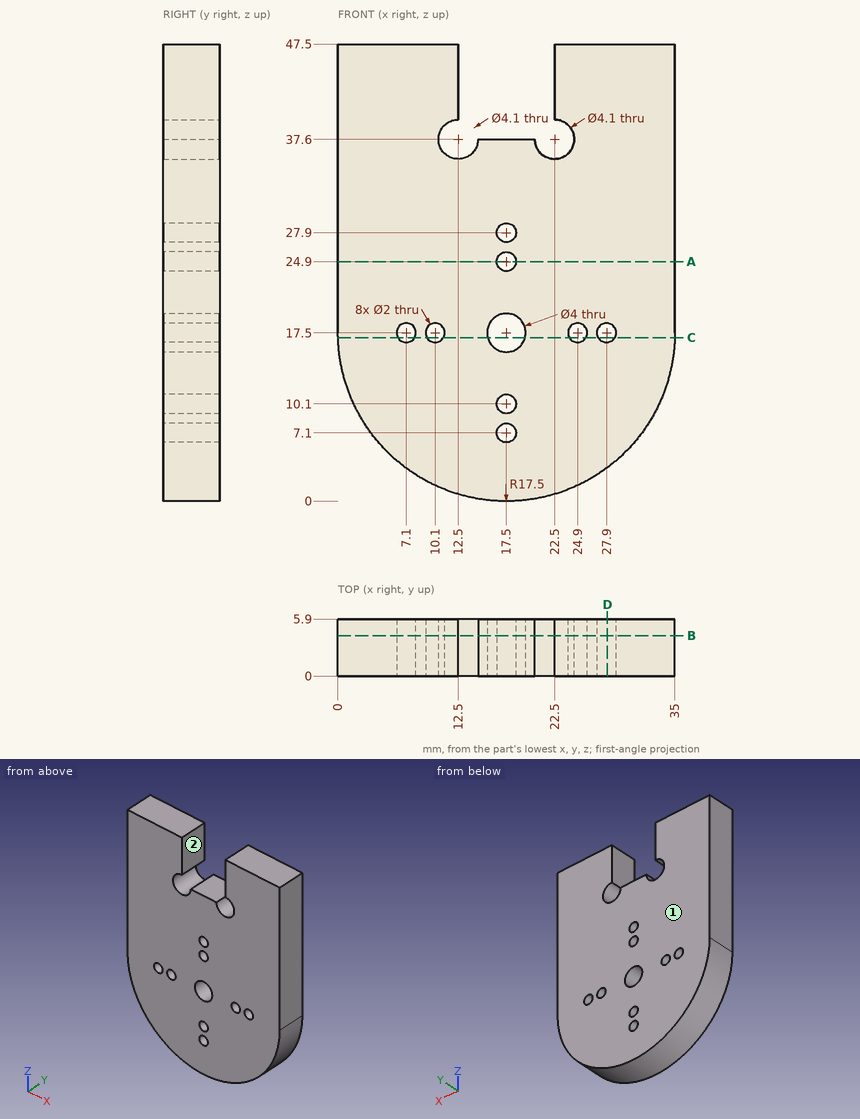
Input: dimensioned drawing with shaded views. Units: mm. Origin: part minimum x, y, z. A direction names the side the tool comes from. Coordinates: 2 decimals unless noted, no trailing zeros. Loops run counter-clockwise (first coordinate to the right, second up) from the corner with the lowest first, then second, coordinate; pieces in that order, holes last. Notation, with made-up numbers: (75, 76.5) -> (87, 76.5) arc R23 ccw to (87, 103.5) -> close; hole circle Ø8 at (27.25, -33). An arc over 180 degrees is marked (long way). One line per item, written item: value. Start each with the question number.
Q1. Section query A-A, the plane z = 24.9. Return the cut outline in (x, y).
Q2. Section query C-C, the plane z = 17. Return the cut outline in (x, y).
Q3. Section query B-B, the plane y = 4.2. Give the number of separate pieces and of enclosed holes in the cut face, and give its area (3 significant figures).
Q4. Line query: line 1 along X through (y, z) = (1.35, 27.9); line 2 along X through (y, z) = (4.5, 18); line 3 along Z through (x, y) = (10.1, 2.6). Output: solid intervals per line, ascending.
Q5. Section query D-D, the plane x = 28. Return the cut outline in (y, z).
Q6. Set-up query: the marked faces 1 and 2. Return all of +Z, -Z, +X, -X, +Y, -Y with unobstructed straight access to the full face (end or side cutting, diameter ignored); none if empty.
Q7. Contact query for flat-ended pins moving along their axis: P1, Ø3, axis at x = 15, y = 1, coming from the +Z side; P2, Ø3.5, axis at x = 22.5, z = 37.6, coming from the -Y side (1 decimal). Output: stop coordinate, or through.
Results:
1. outline: (0, 0) -> (16.5, 0) -> (16.5, 5.9) -> (0, 5.9) -> close; (18.5, 0) -> (35, 0) -> (35, 5.9) -> (18.5, 5.9) -> close
2. outline: (0.01, 0) -> (6.23, 0) -> (6.23, 5.9) -> (0.01, 5.9) -> close; (7.97, 0) -> (9.23, 0) -> (9.23, 5.9) -> (7.97, 5.9) -> close; (10.97, 0) -> (15.56, 0) -> (15.56, 5.9) -> (10.97, 5.9) -> close; (19.44, 0) -> (24.03, 0) -> (24.03, 5.9) -> (19.44, 5.9) -> close; (25.77, 0) -> (27.03, 0) -> (27.03, 5.9) -> (25.77, 5.9) -> close; (28.77, 0) -> (34.99, 0) -> (34.99, 5.9) -> (28.77, 5.9) -> close
3. separate pieces: 1
3. enclosed holes: 9
3. area: 1,370 mm^2
4. line 1: 0 to 16.5, 18.5 to 35
4. line 2: 0 to 6.23, 7.97 to 9.23, 10.97 to 15.56, 19.44 to 24.03, 25.77 to 27.03, 28.77 to 35
4. line 3: 1.64 to 16.5, 18.5 to 47.5
5. outline: (0, 3.5) -> (5.9, 3.5) -> (5.9, 16.51) -> (0, 16.51) -> close; (0, 18.49) -> (5.9, 18.49) -> (5.9, 47.5) -> (0, 47.5) -> close
6. face 1: +Z, -Z, +X, -X, +Y
6. face 2: +Z, +Y, -Y
7. P1: z = 37.6
7. P2: through
